Geometry check sheet. Reference: drawing and pictorial views, mm from the part's lowest x, y, z. A direction names the side the tool comes from. Round coordinates to 2 decimals unless told otherwise and drop trailing zeros. Write each loop counter-clockwise with the first axis right and the second up, starting at its lowest first coordinate (ties: lowest second). Pieces come first, ordered by that corner, then holes.
Item 1: Section check C-C, the plane y = 4.25. Record the cut outline in (x, z).
Item 2: Section check A-A, the plane x = 12.5. Record the cut outline in (y, z).
Item 3: Material ranges on line 1 along Z through (x, y) = (12.5, 5.25); line 2 along Z through (x, y) = (12.5, 6.25) (1 decimal); line 3 along Z through (x, y) = (18.75, 8.5) (1 decimal), recorded low to high.
Item 4: Set-up check for the marked faces 4, 5 and 6: record each of +Z, -Z, +X, -X, +Y, -Y from which the full face is reachable in a straight line by a thin tool's end or side.
Item 5: Depth check by flat-ended pin: pin 1 (2.5 mm diameter, centred on y = 7.5, z = 5, fed in from +X); pin 2 (1.3 mm diameter, centred on x = 5.5, y = 9, fed in from +Z); pin 3 (6 mm diameter, centred on x = 17.5, y = 3, fed in from +Z). Enter the tip coordinate at first touch or a pass-through.
Item 6: Section check B-B, the plane y = 10.25. State how many separate pieces and enclosed holes the cut face has, plus the area to 3 significant figures.
Item 7: Release check for a two-part mould opening along X. For the marked faces 1, 2 and 3 record: pulls with the +X half, pulls with the -X half, needs draft (parallel to the pull), parting line crosses it, or undercut.
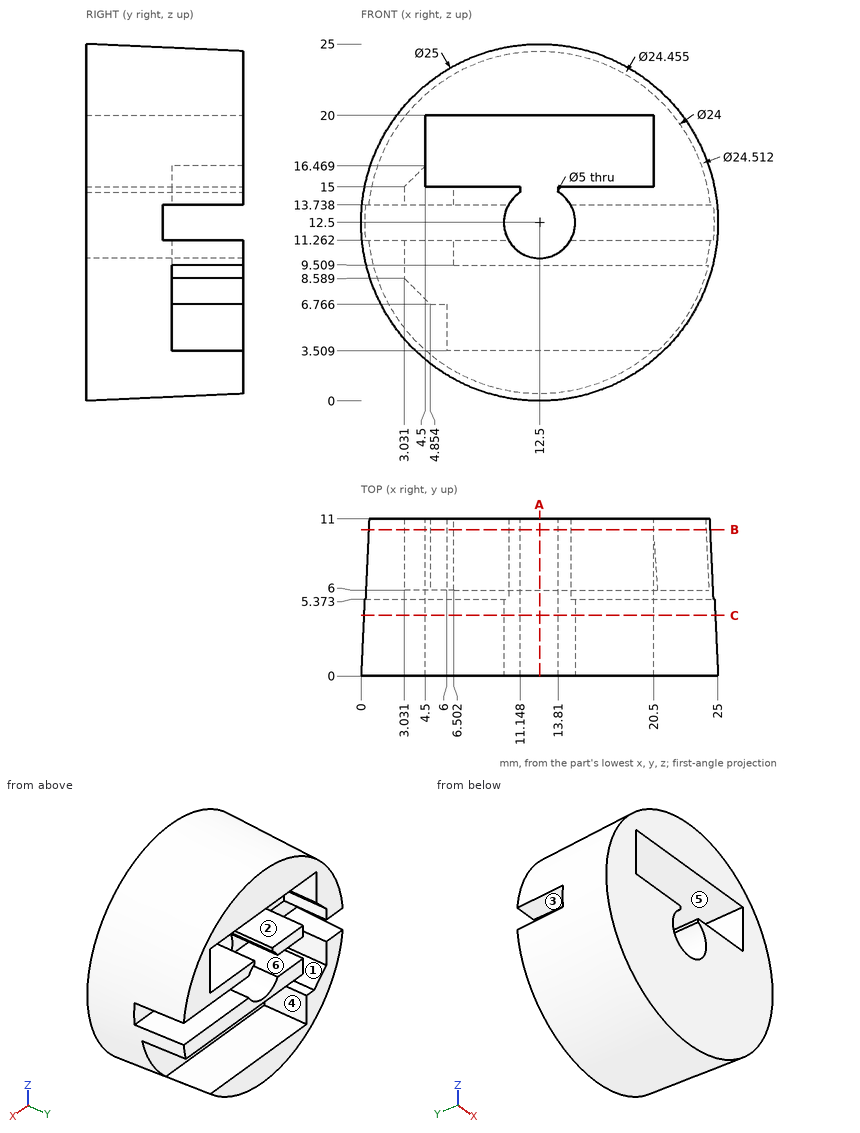
Values found:
1. outline: circle Ø24.61 at (12.5, 12.5); hole (4.5, 15) - (11.15, 15) - (11.15, 14.6) arc R2.5 ccw (long way) to (13.81, 14.63) - (13.81, 15) - (20.5, 15) - (20.5, 20) - (4.5, 20) - close
2. outline: (0, 0) - (11, 0.5) - (11, 3.51) - (6, 3.51) - (6, 9.51) - (11, 9.51) - (11, 10) - (0, 10) - close; (0, 20) - (11, 20) - (11, 24.5) - (0, 25) - close
3. line 1: z = 0.24 to 10, 20 to 24.76
3. line 2: z = 0.3 to 3.5, 9.5 to 10, 20 to 24.7
3. line 3: z = 2.1 to 3.5, 9.5 to 11.3, 13.7 to 15, 20 to 22.9
4. face 4: +X, +Y
4. face 5: +Y, -Y
4. face 6: +X, -X, +Y
5. pin 1: stops at x = 6
5. pin 2: stops at z = 22.79
5. pin 3: stops at z = 24.72
6. separate pieces: 4
6. enclosed holes: 0
6. area: 189 mm2
7. face 1: pulls with the +X half
7. face 2: undercut
7. face 3: needs draft
